from build123d import *

# Parameters (mm, degrees)
SKETCH1_R           = 19.05
SKETCH1_R_2         = 13.335
BOSS_EXTRUDE1_DEPTH = 3.175
SKETCH2_R           = 22.225
SKETCH2_R_2         = 16.03375
BOSS_EXTRUDE2_DEPTH = 3.175
FILLET1_R           = 2.54


with BuildPart() as part:
    # Sketch1 → Boss-Extrude1 (new, symmetric)
    with BuildSketch(Plane.XY):
        Circle(SKETCH1_R)
        Circle(SKETCH1_R_2, mode=Mode.SUBTRACT)
    extrude(amount=BOSS_EXTRUDE1_DEPTH, both=True)

    # Sketch2 → Boss-Extrude2 (add)
    with BuildSketch(Plane.XY.offset(3.175)):
        Circle(SKETCH2_R)
        Circle(SKETCH2_R_2, mode=Mode.SUBTRACT)
    extrude(amount=BOSS_EXTRUDE2_DEPTH)

    # Fillet1
    fillet1_edges = [part.edges().sort_by_distance(p)[0] for p in [
        (-19.05, 0, 3.175),
    ]]
    fillet(fillet1_edges, radius=FILLET1_R)


solid = part.part
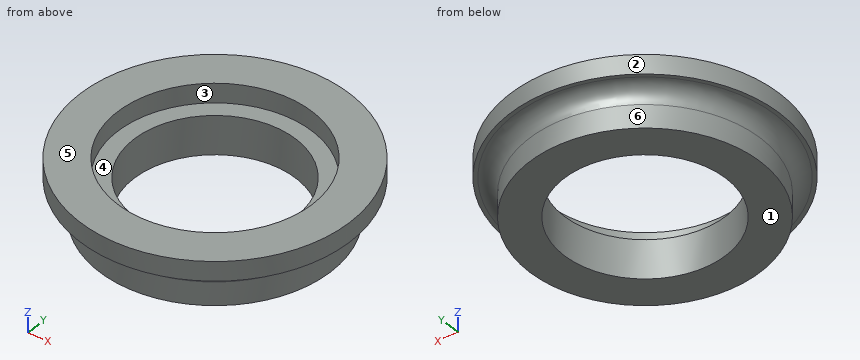
Geometry: final body of the model. Coordinates: model frame, mm. Face numbers are marked on the shaded views. A direction names the side the tool comes from. Give positions to 0.01 mm unless a question says otherwise; leave off trailing zeros. Loops run counter-clockwise (first coordinate to the right, second up) from the corner with the lowest first, then second, coordinate; pieces in that order, holes last. Notation, with made-up numbers: (54.25, 85) - (98.25, 85) arc R34 cw to (98.25, 118) - close; hole circle Ø3 at (59, 43). An arc over 180 degrees is marked (long way). One line per question, with ' | ' between items. Start each with the question number.
(1) Section query A-A on x = 0. Return loops of the section in (y, z) (3 decimals), then the cut area to 3 significant figures.
(2) Contact query for flat-ended pins moving along their axis: pin 1 (1.5 mm diameter, centred on y = -6.5, z = -1, fed in from -X); pin 2 (16 mm diameter, centred on x = 0, y = 0, fed in from -Z); pin 3 (1.5 mm diameter, centred on y = 13, z = 0.5, fed in from +X); pin 4 (5 mm diameter, centred on x = 5, z = -1, fed in from -Y). Output: stop coordinate, or through.
(3) Section query C-C on z = -1. Return loops of the section in (x, y) (3 decimals), then the cut area to 3 significant figures.
(4) Ray query, line 1 (Y direction, x = 0, z = -0.75) (3 decimals); line 2 (Y direction, x = 0, z = 4.7) (3 decimals); line 3 (Z direction, x = -3, y = -15) (3 decimals). Return the intervals inside material, ascending. Write a range as from..to.
(5) Pull-direction query (X, two-part tool) for the marked faces 1, 2, 3 and 4; classes: released by +X, released by -X, zero draft, split by the parting line, or undercut.
(6) Reachability of the marked faces 5 and 6 from +Z, -Z, +X, -X, +Y, -Y: full face, straight path, thin tool, end or side. Return the list, or none.
The answers:
1) outline: (-22.225, 3.175) - (-21.59, 3.175) arc R2.54 cw to (-19.05, 0.635) - (-19.05, -3.175) - (-13.335, -3.175) - (-13.335, 3.175) - (-16.034, 3.175) - (-16.034, 6.35) - (-22.225, 6.35) - close; (13.335, -3.175) - (19.05, -3.175) - (19.05, 0.635) arc R2.54 cw to (21.59, 3.175) - (22.225, 3.175) - (22.225, 6.35) - (16.034, 6.35) - (16.034, 3.175) - (13.335, 3.175) - close | area: 115 mm2
2) pin 1: x = -18.16 | pin 2: through | pin 3: x = 14.59 | pin 4: y = -18.89
3) outline: circle Ø38.1 at (0, 0); hole circle Ø26.67 at (0, 0) | area: 581 mm2
4) line 1: -19.05..-13.335, 13.335..19.05 | line 2: -22.225..-16.034, 16.034..22.225 | line 3: -3.175..3.175
5) face 1: zero draft | face 2: split by the parting line | face 3: undercut | face 4: undercut
6) face 5: +Z, +X, -X, +Y, -Y | face 6: -Z
